```python
from build123d import *

# Parameters (mm, degrees)
SKETCH_1_W          = 150
SKETCH_1_H          = 150
EXTRUDE_2_DEPTH     = 5
SKETCH_1_3_W        = 150
SKETCH_1_3_H        = 150
SKETCH_1_3_W_2      = 140
SKETCH_1_3_H_2      = 140
EXTRUDE_3_DEPTH     = 100
SKETCH_3_W          = 130
SKETCH_3_H          = 8.266043605
CUT_EXTRUDE_1_DEPTH = 5


with BuildPart() as part:
    # 草图1 → 凸台-拉伸2 (new body)
    with BuildSketch(Plane(origin=(0, 0, 0), x_dir=(1, 0, 0), z_dir=(0, 1, 0))):
        with Locations((-75, -75)):
            Rectangle(SKETCH_1_W, SKETCH_1_H)
    extrude(amount=EXTRUDE_2_DEPTH)

    # 草图1<3> → 凸台-拉伸3 (add)
    with BuildSketch(Plane(origin=(0, 0, 0), x_dir=(1, 0, 0), z_dir=(0, 1, 0))):
        with Locations((-75, -75)):
            Rectangle(SKETCH_1_3_W, SKETCH_1_3_H)
        with Locations((-75, -75)):
            Rectangle(SKETCH_1_3_W_2, SKETCH_1_3_H_2, mode=Mode.SUBTRACT)
    extrude(amount=-EXTRUDE_3_DEPTH)

    # 草图3 → 切除-拉伸1 (cut)
    with BuildSketch(Plane.XY.offset(150)):
        with Locations((-75, -95.866978198)):
            Rectangle(SKETCH_3_W, SKETCH_3_H)
    extrude(amount=-CUT_EXTRUDE_1_DEPTH, mode=Mode.SUBTRACT)


solid = part.part
```
Here's how the part is built. I have some questions about the finished solid (model axes, mm). A direction names the side the tool comes from. Give positions to 0.01 mm unless a question says otherwise; leave off trailing zeros. Loops run counter-clockwise (first coordinate to the right, second up) from the corner with the lowest first, then second, coordinate; pieces in that order, holes last. Notation, with made-up numbers: M 89.5,71 L 126.5,71 A25 cw 126.5,102 Z; hole C -3,30 d6. An arc over 180 degrees is marked long. Return JSON: item names as keys, results as strings.
Item 1: On a 3-axis mill with a long thin cutter (end or side, diameter ignored), from which of +Z, -Z, +X, -X, +Y, -Y can I reach the whole of each face in a straight line? I mean faces 4 (the flat face through (-140, -96, 148)), 5 (the flat face through (-75, -100, 2)), 6 (the flat face through (-76, 0, 74)). Say none if no direction works.
A:
{"face 4": "+Z, -Y", "face 5": "+Z, -Z, +X, -X, -Y", "face 6": "-Y"}
Item 2: I'm going to push flat-ended pins straight in: pin 1 Ø10 at (x, z) = (-134.5, 114) entering from -Y; pin 2 Ø4 at (x, z) = (-79, 148) entering from -Y. Where does each tip first touch, or does it pass through?
A:
{"pin 1": "stops at y = 0", "pin 2": "stops at y = -91.73"}
Item 3: Please list where these lines run through material, in increasing order: line 1 (Z direction, x = -125, y = -4); line 2 (X direction, y = -26, z = 74); line 3 (Y direction, x = -18.5, z = 137).
A:
{"line 1": "z = 0 to 5, 145 to 150", "line 2": "x = -150 to -145, -5 to 0", "line 3": "y = 0 to 5"}
Item 4: Imagine slicing it at C-C on x = -135. List the corners of the cut face in (y, z) for me.
A:
{"outline": "M -100,0 L 5,0 L 5,150 L -91.73,150 L -91.73,145 L 0,145 L 0,5 L -100,5 Z"}
Item 5: Thinking about a two-plate mould opening in X: for faces 1 (the flat face through (-150, -47, 76)), 2 (the flat face through (-76, -91.734, 148)), 3 (the flat face through (-76, 5, 74)), which applies, released by +X, released by -X, zero draft, split by the parting line, or undercut?
A:
{"face 1": "released by -X", "face 2": "undercut", "face 3": "zero draft"}
Item 6: Imagine slicing it at A-A on y = -5.5. List the corners of the cut face in (x, z) for me, then the cut area to 3 significant figures.
A:
{"outline": "M -150,0 L 0,0 L 0,150 L -150,150 Z; hole M -145,5 L -5,5 L -5,145 L -145,145 Z", "area": "2,900 mm^2"}
Item 7: Imagine slicing it at B-B on z = 58. List the corners of the cut face in (x, y) for me.
A:
{"outline": "M -150,-100 L -145,-100 L -145,0 L -5,0 L -5,-100 L 0,-100 L 0,5 L -150,5 Z"}
